Could you check a few things on this drawing? It's one solid part, dimensions in mm from its lowest x, y, z. A direction names the side the tool comes from. Round coordinates to 2 decimals unless told otherwise and drop trailing zeros. Loops run counter-clockwise (first coordinate to the right, second up) from the corner with the lowest first, then second, coordinate; pieces in that order, holes last. Notation, with made-up numbers: (-0.5, 23.5) -> (50.5, 23.5) arc R20 ccw to (50.5, 44.5) -> close; hole circle Ø1 at (73, -14). An arc over 180 degrees is marked (long way). Write each question's results on one line, items separated by ' | '.
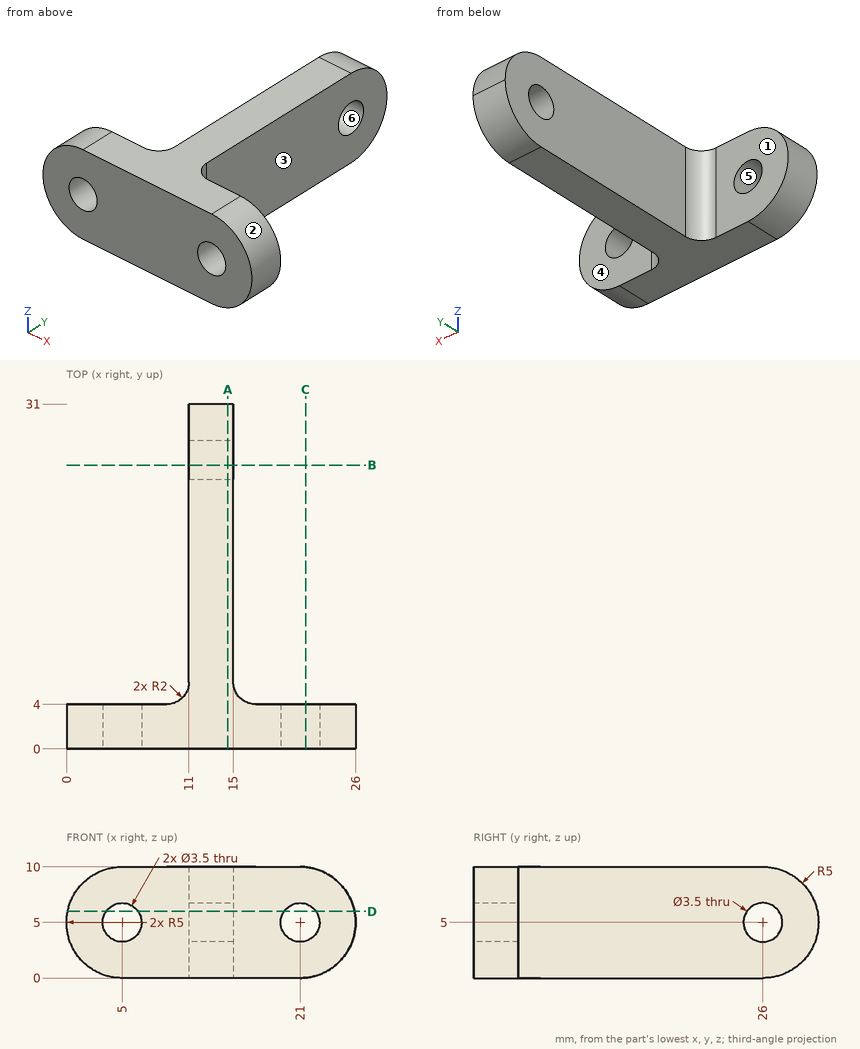
1) I want a section at B-B, the plane y = 25.5. Write out the boundary of the cut face in (x, z), plus the area to 3 significant figures.
Model answer:
outline: (11, 0) -> (15, 0) -> (15, 3.32) -> (11, 3.32) -> close; (11, 6.68) -> (15, 6.68) -> (15, 10) -> (11, 10) -> close | area: 26.6 mm2
2) For the marked faces 1, 2 and 3, which set-ups out of +Z, -Z, +X, -X, +Y, -Y let a thin tool reach every point of the face, with its end or its side?
Model answer:
face 1: +Z, -Z, -X, +Y | face 2: +X, +Y, -Y | face 3: +Z, -Z, +X, +Y
3) I want a section at A-A, the plane x = 14.5. Write out the boundary of the cut face in (y, z), plus the area to 3 significant figures.
Model answer:
outline: (0, 0) -> (26, 0) arc R5 ccw to (26, 10) -> (0, 10) -> close; hole circle Ø3.5 at (26, 5) | area: 290 mm2
4) If we mould it in two halves opening along Y, with no side actions, what happens to the marked faces 4, 5 and 6? For each: released by +Y, released by -Y, zero draft, split by the parting line, or undercut.
Model answer:
face 4: released by +Y | face 5: zero draft | face 6: undercut
5) I'm going to push flat-ended pins straight in: pin 1 (4.5 mm diameter, centred on x = 6, z = 2.5, fed in from +Y); pin 2 (3 mm diameter, centred on y = 22.5, z = 7.5, fed in from -X); pin 3 (3 mm diameter, centred on y = 27.5, z = 9, fed in from +X); pin 4 (2 mm diameter, centred on x = 5, z = 5, fed in from +Y). Where does each tip first touch, or does it pass through?
Model answer:
pin 1: stops at y = 4 | pin 2: stops at x = 11 | pin 3: stops at x = 15 | pin 4: passes through
6) I want a section at D-D, the plane z = 6. Write out the boundary of the cut face in (x, y).
Model answer:
outline: (0.1, 0) -> (3.56, 0) -> (3.56, 4) -> (0.1, 4) -> close; (6.44, 0) -> (19.56, 0) -> (19.56, 4) -> (17, 4) arc R2 cw to (15, 6) -> (15, 24.56) -> (11, 24.56) -> (11, 6) arc R2 cw to (9, 4) -> (6.44, 4) -> close; (11, 27.44) -> (15, 27.44) -> (15, 30.9) -> (11, 30.9) -> close; (22.44, 0) -> (25.9, 0) -> (25.9, 4) -> (22.44, 4) -> close
7) I need wall thicknesses on line 1 (X direction, y = 2.3, z = 5); line 2 (Y direction, x = 7.25, z = 9.75); line 3 (X direction, y = 20, z = 3.5). Which ranges of each line are inside material? Lowest first, please.
Model answer:
line 1: x = 0 to 3.25, 6.75 to 19.25, 22.75 to 26 | line 2: y = 0 to 4 | line 3: x = 11 to 15
8) I want a section at C-C, the plane x = 21.5. Write out the boundary of the cut face in (y, z).
Model answer:
outline: (0, 0.03) -> (4, 0.03) -> (4, 3.32) -> (0, 3.32) -> close; (0, 6.68) -> (4, 6.68) -> (4, 9.97) -> (0, 9.97) -> close
